Verification items for the finished model (mm, model axes). A direction names the side the tool comes from. Coordinates: 2 decimals unless noted, no trailing zeros. Return JSON: item names as keys, results as strings.
```python
from build123d import *

# Parameters (mm, degrees)
F0_R      = 225
F0_R_2    = 120
F1_DEPTH  = 5
F2_R      = 2.49999
F3_R      = 195
F3_R_2    = 120
F4_DEPTH  = 30
F5_R      = 20
F6_DEPTH  = 15
F8_DEPTH  = 35.001
F10_D     = 6
F10_DEPTH = 20
F10_TIP   = 1.8025818571
F12_D     = 6
F12_DEPTH = 20
F12_TIP   = 1.8025818571


# Not quite as in the source:
# - a fillet or chamfer is up to 0.001 mm smaller than in the source, because OpenCascade refuses the exact size
# - a feature names something its author has since deleted; it is built from what else it names


with BuildPart() as f1:
    # F0 (on Top) → F1 (new body)
    with BuildSketch(Plane.XY):
        Circle(F0_R)
        Circle(F0_R_2, mode=Mode.SUBTRACT)
    extrude(amount=F1_DEPTH)

    # F2 (radius 2.5 in the source; OpenCascade refuses exactly that, so slightly less here)
    f2_edges = [f1.edges().sort_by_distance(p)[0] for p in [
        (-225, 0, 5),
        (-225, 0, 0),
    ]]
    fillet(f2_edges, radius=F2_R)

    # F3 (on face) → F4 (join)
    with BuildSketch(Plane.XY.offset(5)):
        Circle(F3_R)
        Circle(F3_R_2, mode=Mode.SUBTRACT)
    extrude(amount=F4_DEPTH)

    # F5 (on face) → F6 (cut)
    with BuildSketch(Plane(origin=(0, 0, 0), x_dir=(1, 0, 0), z_dir=(0, 0, -1))):
        with BuildLine():
            ThreePointArc((20, 160), (-14.1421356237, 174.1421356237), (0, 140))
            ThreePointArc((0, 140), (14.1421356237, 145.8578643763), (20, 160))
        make_face()
        with Locations((138.5640646055, -80)):
            Circle(F5_R)
        with Locations((-138.5640646055, -80)):
            Circle(F5_R)
    extrude(amount=-F6_DEPTH, mode=Mode.SUBTRACT)

    # F7 (on face) → F8 (cut, through all)
    with BuildSketch(Plane.XY.offset(35)):
        with BuildLine():
            Line((0, 125), (0, 120))
            ThreePointArc((0, 120), (3.501490936, 119.9489039601), (7, 119.7956593538))
            Line((7, 119.7956593538), (7, 125))
            Line((7, 125), (0, 125))
        make_face()
        with BuildLine():
            ThreePointArc((-7, 119.7956593538), (-3.501490936, 119.9489039601), (0, 120))
            Line((0, 120), (0, 125))
            Line((0, 125), (-7, 125))
            Line((-7, 125), (-7, 119.7956593538))
        make_face()
        with BuildLine():
            Line((7, -125), (7, -119.7956593538))
            ThreePointArc((7, -119.7956593538), (3.501490936, -119.9489039601), (0, -120))
            Line((0, -120), (0, -125))
            Line((0, -125), (7, -125))
        make_face()
        with BuildLine():
            ThreePointArc((0, -120), (-3.501490936, -119.9489039601), (-7, -119.7956593538))
            Line((-7, -119.7956593538), (-7, -125))
            Line((-7, -125), (0, -125))
            Line((0, -125), (0, -120))
        make_face()
    extrude(amount=-F8_DEPTH, mode=Mode.SUBTRACT)

    # F10 (one way)
    with BuildSketch(Plane(origin=(0, -125, 0), x_dir=(-1, 0, 0), z_dir=(0, 1, 0))):
        with Locations((0, 20)):
            Circle(F10_D / 2)
    extrude(amount=-F10_DEPTH, mode=Mode.SUBTRACT)
    with Locations(Plane(origin=(0, -125, 0), x_dir=(-1, 0, 0), z_dir=(0, 1, 0))):
        with Locations((0, 20)):
            with Locations((0, 0, -(F10_DEPTH + F10_TIP / 2))):  # 118° drill point
                Cone(0, F10_D / 2, F10_TIP, mode=Mode.SUBTRACT)

    # F12 (one way)
    with BuildSketch(Plane.XZ.offset(-125)):
        with Locations((0, 20)):
            Circle(F12_D / 2)
    extrude(amount=-F12_DEPTH, mode=Mode.SUBTRACT)
    with Locations(Plane.XZ.offset(-125)):
        with Locations((0, 20)):
            with Locations((0, 0, -(F12_DEPTH + F12_TIP / 2))):  # 118° drill point
                Cone(0, F12_D / 2, F12_TIP, mode=Mode.SUBTRACT)


solid = f1.part
```
Q1. Go/stop test with flat-tipped pins: pin 1 (10 mm diameter, centred on x = -167.5, z = 29, fed in from +Y); pin 2 (5.5 mm diameter, centred on y = 123, z = 14.5, fed in from +X); pin 3 (3 mm diameter, centred on x = 62.5, z = 13, fed in from -Y). Record where each tip stops, or that it passes through.
Values:
{"pin 1": "y = 107.79", "pin 2": "x = 153.51", "pin 3": "y = -185.21"}
Q2. Tool access check on faces 5 (the face through (96, -96, 0)), 6 (the face through (-139, 80, 15)), 7 (the face through (-119.973, 2.541, 17.255)). Record the directions out of +Z, -Z, +X, -X, +Y, -Y that give a thin tool (end or side, any length) a straight path to the whole face; none if there is none.
Values:
{"face 5": "-Z, +X, -X, +Y, -Y", "face 6": "-Z", "face 7": "+Z, -Z"}
Q3. Draft check along Y on faces 1 (the face through (3, 125, 18)), 2 (the face through (-1, -197, 5)), 3 (the face through (-154.75, -118.65, 19.79)), 4 (the face through (119.973, -2.541, 17.255)). Enter one of: pulls with the +Y half, pulls with the -Y half, needs draft (parallel to the pull), parting line crosses it, or undercut.
Values:
{"face 1": "undercut", "face 2": "needs draft", "face 3": "parting line crosses it", "face 4": "undercut"}
Q4. Material ranges on line 1 along Z through (x, y) = (0, -131.75); line 2 along X through (y, z) = (-59.5, 21); line 3 along Z through (x, y) = (-187, 95), recorded low to high.
Values:
{"line 1": "0 to 17, 23 to 35", "line 2": "-185.7 to -104.21, 104.21 to 185.7", "line 3": "0 to 5"}
